Here's how the part is built. I have some questions about the finished solid (model axes, mm). A direction names the side the tool comes from. Give positions to 0.01 mm unless a question says otherwise; leave off trailing zeros. Write each loop counter-clockwise with the first axis right and the second up, starting at its lowest first coordinate (ties: lowest second). Pieces come first, ordered by that corner, then holes. Notation, with made-up numbers: (-31.5, 37.25) - (-17.5, 37.25) arc R8 cw to (-17.5, 44.25) - close; hole circle Ø6 at (85, 69.5). An arc over 180 degrees is marked (long way). Use a Markdown table: item, result.
```python
from build123d import *

# Parameters (mm, degrees)
SKETCH1_R           = 2.25
BOSS_EXTRUDE1_DEPTH = 2


with BuildPart() as part:
    # Sketch1 → Boss-Extrude1 (new, symmetric)
    with BuildSketch(Plane.XY):
        with BuildLine():
            Line((0, 10), (175, 10))
            ThreePointArc((175, 10), (185, 0), (175, -10))
            Line((175, -10), (0, -10))
            ThreePointArc((0, -10), (-5.00000204, -8.66025286), (-8.660256393, -4.99999592))
            Line((-8.660256393, -4.99999592), (-30, -5))
            ThreePointArc((-30, -5), (-35, 0), (-30, 5))
            Line((-30, 5), (-8.660256485, 4.999995761))
            ThreePointArc((-8.660256485, 4.999995761), (-5.000002119, 8.660252814), (0, 10))
        make_face()
        Circle(SKETCH1_R, mode=Mode.SUBTRACT)
        with Locations((-30, 0)):
            Circle(SKETCH1_R, mode=Mode.SUBTRACT)
        with Locations((175, 0)):
            Circle(SKETCH1_R, mode=Mode.SUBTRACT)
    extrude(amount=BOSS_EXTRUDE1_DEPTH, both=True)


solid = part.part
```
Item 1: If we section it at B-B, the plane z = -0.9: Write out the boundary of the cut face in (x, y), plus the area to 3 significant figures.
Values:
| item | result |
|---|---|
| outline | (-30, -5) - (-8.66, -5) arc R10 ccw to (0, -10) - (175, -10) arc R10 ccw to (175, 10) - (0, 10) arc R10 ccw to (-8.66, 5) - (-30, 5) arc R5 ccw to start; hole circle Ø4.5 at (-30, 0); hole circle Ø4.5 at (0, 0); hole circle Ø4.5 at (175, 0) |
| area | 4,010 mm2 |
Item 2: Thinking about a two-plate mould opening in X: for faces 4 (the flat face through (77, 0, 2)), 5 (the cylindrical face through (177.08, -0.86, -0.03)), 6 (the cylindrical face through (-4.936, -8.697, 0.028)), which applies, +X half, -X half, draft (parallel to the pull), parting line (faces both ways), or undercut?
Values:
| item | result |
|---|---|
| face 4 | draft |
| face 5 | undercut |
| face 6 | -X half |
Item 3: Will this pin go through, and if not, where does the flat tip stop? pin 1 Ø7 at (x, y) = (-30, 0) entering from -Z.
Values:
| item | result |
|---|---|
| pin 1 | stops at z = -2 |
Item 4: If we section it at C-C, the plane x = -16.5: Write out the boundary of the cut face in (y, z), plus the area to 3 significant figures.
Values:
| item | result |
|---|---|
| outline | (-5, -2) - (5, -2) - (5, 2) - (-5, 2) - close |
| area | 40.0 mm2 |
Item 5: I need wall thicknesses on line 1 along Y through (x, z) = (-30, -1.2); line 2 along X through (y, z) = (1.75, -1.7); line 3 along Y through (x, z) = (175, 1). Which ranges of each line are inside material? Lowest first, please. Write a range as [from, to].
Values:
| item | result |
|---|---|
| line 1 | y = [-5, -2.25], [2.25, 5] |
| line 2 | x = [-34.68, -31.41], [-28.59, -1.41], [1.41, 173.59], [176.41, 184.85] |
| line 3 | y = [-10, -2.25], [2.25, 10] |
Item 6: If we section it at A-A, the plane y = 0: Write out the boundary of the cut face in (x, z).
Values:
| item | result |
|---|---|
| outline | (-35, -2) - (-32.25, -2) - (-32.25, 2) - (-35, 2) - close; (-27.75, -2) - (-2.25, -2) - (-2.25, 2) - (-27.75, 2) - close; (2.25, -2) - (172.75, -2) - (172.75, 2) - (2.25, 2) - close; (177.25, -2) - (185, -2) - (185, 2) - (177.25, 2) - close |
Item 7: For faces 1 (the flat face through (77, 0, -2)), 2 (the flat face through (-19, 5, 0)), 3 (the flat face through (-19, -5, 0)), which set-ups out of +Z, -Z, +X, -X, +Y, -Y let a thin tool reach every point of the face, with its end or its side?
Values:
| item | result |
|---|---|
| face 1 | -Z, +X, -X, +Y, -Y |
| face 2 | +Z, -Z, -X, +Y |
| face 3 | +Z, -Z, -X, -Y |
